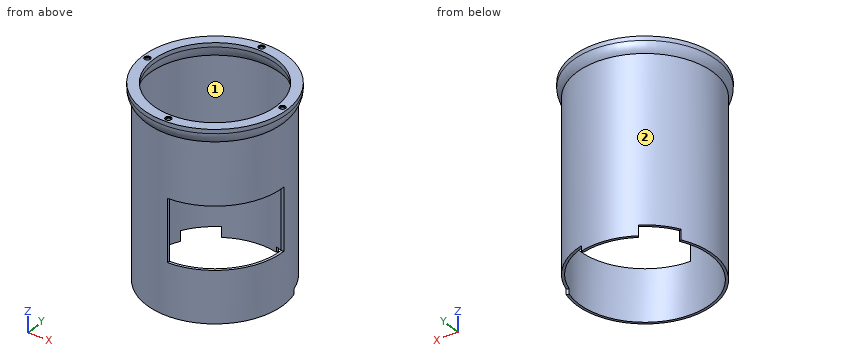
from build123d import *

# Parameters (mm, degrees)
SKIZZE1_R                       = 70
SKIZZE1_R_2                     = 60
AUFSATZ_LINEAR_AUSTRAGEN1_DEPTH = 14
AUFSATZ_LINEAR_START            = -14
SKIZZE10_R                      = 66.25
SKIZZE10_R_2                    = 63.75
AUFSATZ_LINEAR_AUSTRAGEN2_DEPTH = 170
SCHNITT_LINEAR_START            = -74
SCHNITT_LINEAR_AUSTRAGEN1_DEPTH = 60
SCHNITT_LINEAR_START_2          = -174
SCHNITT_LINEAR_AUSTRAGEN3_DEPTH = 10
SCHNITT_LINEAR_START_3          = -179
SCHNITT_LINEAR_AUSTRAGEN4_DEPTH = 5
SKIZZE3_R                       = 2
SCHNITT_LINEAR_AUSTRAGEN5_DEPTH = 7
SKIZZE9_R                       = 3
SCHNITT_LINEAR_AUSTRAGEN6_DEPTH = 1
VERRUNDUNG4_R                   = 15
VERRUNDUNG5_R                   = 15


with BuildPart() as part:
    # Skizze1 → Aufsatz-Linear austragen1 (new body)
    with BuildSketch(Plane(origin=(0, 0, 0), x_dir=(0, 1, 0), z_dir=(0, 0, 1))):
        with Locations(Location((0, 0, 0), (0, 0, 270))):
            Circle(SKIZZE1_R)
        with Locations(Location((0, 0, 0), (0, 0, 270))):
            Circle(SKIZZE1_R_2, mode=Mode.SUBTRACT)
    extrude(amount=-AUFSATZ_LINEAR_AUSTRAGEN1_DEPTH)

    # Skizze10 → Aufsatz-Linear austragen2 (add)
    with BuildSketch(Plane.XY.offset(AUFSATZ_LINEAR_START)):
        Circle(SKIZZE10_R)
        Circle(SKIZZE10_R_2, mode=Mode.SUBTRACT)
    extrude(amount=-AUFSATZ_LINEAR_AUSTRAGEN2_DEPTH)

    # Skizze4 → Schnitt-Linear austragen1 (cut)
    with BuildSketch(Plane(origin=(0, 0, 0), x_dir=(0, 1, 0), z_dir=(0, 0, 1)).offset(SCHNITT_LINEAR_START)):
        with BuildLine():
            Line((-70, 0), (-60, 0))
            ThreePointArc((-60, 0), (-42.426406871, -42.426406871), (0, -60))
            Line((0, -60), (0, -70))
            ThreePointArc((0, -70), (-49.497474683, -49.497474683), (-70, 0))
        make_face()
    extrude(amount=-SCHNITT_LINEAR_AUSTRAGEN1_DEPTH, mode=Mode.SUBTRACT)

    # Skizze5 → Schnitt-Linear austragen3 (cut)
    with BuildSketch(Plane(origin=(0, 0, 0), x_dir=(0, 1, 0), z_dir=(0, 0, 1)).offset(SCHNITT_LINEAR_START_2)):
        with BuildLine():
            Line((30, 51.961524227), (35, 60.621778265))
            ThreePointArc((35, 60.621778265), (49.497474683, 49.497474683), (60.621778265, 35))
            Line((60.621778265, 35), (51.961524227, 30))
            ThreePointArc((51.961524227, 30), (42.426406871, 42.426406871), (30, 51.961524227))
        make_face()
    extrude(amount=-SCHNITT_LINEAR_AUSTRAGEN3_DEPTH, mode=Mode.SUBTRACT)

    # Skizze6 → Schnitt-Linear austragen4 (cut)
    with BuildSketch(Plane(origin=(0, 0, 0), x_dir=(0, 1, 0), z_dir=(0, 0, 1)).offset(SCHNITT_LINEAR_START_3)):
        with BuildLine():
            Line((57.955549577, -15.529142706), (67.61480784, -18.117333157))
            ThreePointArc((67.61480784, -18.117333157), (49.497474683, -49.497474683), (18.117333157, -67.61480784))
            Line((18.117333157, -67.61480784), (15.529142706, -57.955549577))
            ThreePointArc((15.529142706, -57.955549577), (42.426406871, -42.426406871), (57.955549577, -15.529142706))
        make_face()
    extrude(amount=-SCHNITT_LINEAR_AUSTRAGEN4_DEPTH, mode=Mode.SUBTRACT)

    # Skizze3 → Schnitt-Linear austragen5 (cut)
    with BuildSketch(Plane(origin=(0, 0, 0), x_dir=(0, 1, 0), z_dir=(0, 0, 1))):
        with Locations(Location((-65, 0, 0), (0, 0, 270))):
            Circle(SKIZZE3_R)
        with Locations(Location((0, 65, 0), (0, 0, 270))):
            Circle(SKIZZE3_R)
        with Locations(Location((65, 0, 0), (0, 0, 270))):
            Circle(SKIZZE3_R)
        with Locations(Location((0, -65, 0), (0, 0, 270))):
            Circle(SKIZZE3_R)
    extrude(amount=-SCHNITT_LINEAR_AUSTRAGEN5_DEPTH, mode=Mode.SUBTRACT)

    # Skizze9 → Schnitt-Linear austragen6 (cut)
    with BuildSketch(Plane(origin=(0, 0, 0), x_dir=(0, 1, 0), z_dir=(0, 0, 1))):
        with Locations(Location((0, 65, 0), (0, 0, 270))):
            Circle(SKIZZE9_R)
        with Locations(Location((65, 0, 0), (0, 0, 270))):
            Circle(SKIZZE9_R)
        with Locations(Location((0, -65, 0), (0, 0, 270))):
            Circle(SKIZZE9_R)
        with Locations(Location((-65, 0, 0), (0, 0, 270))):
            Circle(SKIZZE9_R)
    extrude(amount=-SCHNITT_LINEAR_AUSTRAGEN6_DEPTH, mode=Mode.SUBTRACT)

    # Verrundung4
    # the kernel refuses this fillet: 15 mm, written as the material it takes off along each edge
    with BuildSketch(Plane(origin=(0, 0, -14), x_dir=(1, 0, 0), z_dir=(0, -1, 0))) as verrundung4_piece_1:
        with BuildLine():
            CenterArc((75, 9.921567416), VERRUNDUNG4_R, 180, 41.409622109)
            Line((63.75, 0), (60, 0))
            Line((60, 0), (60, 9.921567416))
        make_face()
    revolve(axis=Axis((0, 0, -14), (0, 0, 1)), mode=Mode.SUBTRACT)

    # Verrundung5
    # the kernel refuses this fillet: 15 mm, written as the material it takes off along each edge
    with BuildSketch(Plane(origin=(0, 0, -14), x_dir=(1, 0, 0), z_dir=(0, -1, 0))) as verrundung5_piece_1:
        with BuildLine():
            CenterArc((55, 9.921567416), VERRUNDUNG5_R, 318.590377891, 41.409622109)
            Line((66.25, 0), (70, 0))
            Line((70, 0), (70, 9.921567416))
        make_face()
    revolve(axis=Axis((0, 0, -14), (0, 0, 1)), mode=Mode.SUBTRACT)


solid = part.part
Here's how the part is built. I have some questions about the finished solid (model axes, mm). Face numbers are marked on the shaded views. Round coordinates to 2 decimals unless told otherwise and drop trailing zeros. Write each loop counter-clockwise with the first axis right and the second up, starting at its lowest first coordinate (ties: lowest second). Pieces come first, ordered by that corner, then holes.
1. Will these pins go through, and if not, where does the flat tip stop? pin 1 Ø10 at (x, y) = (-37.5, -42.5) entering from +Z; pin 2 Ø2 at (x, z) = (65, -112) entering from -Y; pin 3 Ø8 at (x, z) = (16, -55.5) entering from -Y; pin 4 Ø12 at (y, z) = (42.5, -77) entering from -X.
2. If we mould it in two halves opening along X, with no side actions, what happens to the marked faces 1 and 2? For each: released by +X, released by -X, zero draft, split by the parting line, or undercut.
3. I need wall thicknesses on L1, parallel to Y at x = 0, z = -3.9; L2, parallel to Y at x = 0, z = -0.55; L3, parallel to Y at x = -35, z = -122. Which ranges of each line are inside material? Lowest first, please.
4. Suppose I cut it at B-B (y = -22.5). State how many separate pieces and enclosed holes the cut face has, and give its area (3 significant figures).
5. Suppose I cut it at C-C (z = -113). List the corners of the cut face in (x, y) for me.
6. Suppose I cut it at A-A (z = -20.5). List the corners of the cut face in (x, y) for me, and give its area (3 significant figures).
Answer sheet:
1. pin 1: stops at z = 0
1. pin 2: stops at y = 0
1. pin 3: stops at y = -65.15
1. pin 4: stops at x = -55.29
2. face 1: undercut
2. face 2: split by the parting line
3. L1: y = -70 to -67, -63 to -60, 60 to 63, 67 to 70
3. L2: y = -70 to -68, -62 to -60, 60 to 62, 68 to 70
3. L3: y = -56.25 to -53.28, 53.28 to 56.25
4. separate pieces: 3
4. enclosed holes: 0
4. area: 995 mm2
5. outline: (0, -66.25) - (0, -63.75) arc R63.75 cw (long way) to (63.75, 0) - (66.25, 0) arc R66.25 ccw (long way) to start
6. outline: circle Ø132.5 at (0, 0); hole circle Ø127.5 at (0, 0)
6. area: 1,020 mm2
